from build123d import *

# Parameters (mm, degrees)
SKETCH1_W           = 40
SKETCH1_H           = 40
BOSS_EXTRUDE1_DEPTH = 5
SKETCH2_W           = 60
SKETCH2_H           = 60
BOSS_EXTRUDE2_DEPTH = 5
SKETCH3_R           = 7.5
BOSS_EXTRUDE3_DEPTH = 30
SKETCH4_W           = 30
SKETCH4_H           = 24
BOSS_EXTRUDE5_DEPTH = 10
FILLET1_R           = 5


with BuildPart() as part:
    # Sketch1 → Boss-Extrude1 (new body)
    with BuildSketch(Plane(origin=(0, 0, 0), x_dir=(1, 0, 0), z_dir=(0, 1, 0))):
        with Locations((20, 20)):
            Rectangle(SKETCH1_W, SKETCH1_H)
    extrude(amount=BOSS_EXTRUDE1_DEPTH)

    # Sketch2 → Boss-Extrude2 (add)
    with BuildSketch(Plane(origin=(0, 0, 0), x_dir=(-1, 0, 0), z_dir=(0, -1, 0))):
        with Locations((-20, 20)):
            Rectangle(SKETCH2_W, SKETCH2_H)
    extrude(amount=BOSS_EXTRUDE2_DEPTH)

    # Sketch3 → Boss-Extrude3 (add)
    with BuildSketch(Plane(origin=(0, -5, 0), x_dir=(-1, 0, 0), z_dir=(0, -1, 0))):
        with Locations(Location((-20, 5, 0), (0, 0, 90))):
            Circle(SKETCH3_R)
        with Locations(Location((-20, 35, 0), (0, 0, 90))):
            Circle(SKETCH3_R)
    extrude(amount=BOSS_EXTRUDE3_DEPTH)

    # Sketch4 → Boss-Extrude5 (add)
    with BuildSketch(Plane(origin=(0, -35, 0), x_dir=(-1, 0, 0), z_dir=(0, -1, 0))):
        with Locations((-25, 5)):
            Rectangle(SKETCH4_W, SKETCH4_H)
        with Locations((-25, 35)):
            Rectangle(SKETCH4_W, SKETCH4_H)
    extrude(amount=-BOSS_EXTRUDE5_DEPTH)

    # Fillet1
    fillet1_edges = [part.edges().sort_by_distance(p)[0] for p in [
        (40, -30, 7),
        (40, -30, -17),
        (10, -30, -17),
        (10, -30, 7),
        (40, -30, -23),
        (40, -30, -47),
        (10, -30, -47),
        (10, -30, -23),
    ]]
    fillet(fillet1_edges, radius=FILLET1_R)


solid = part.part
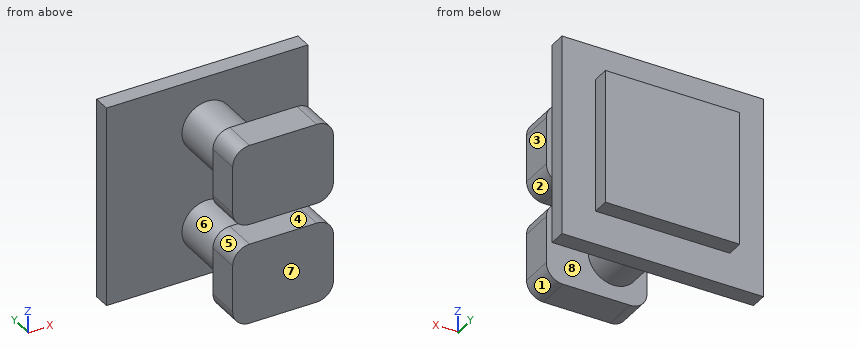
Design review of the part built by this model. Coordinates are the model's own, in mm. Face numbers are marked on the shaded views. A direction names the side the tool comes from. Round coordinates to 2 decimals unless told otherwise and drop trailing zeros. Write each loop counter-clockwise with the first axis right and the second up, starting at its lowest first coordinate (ties: lowest second). Pieces come first, ordered by that corner, then holes. Notation, with made-up numbers: (15.5, 7) -> (40.5, 7) arc R32 cw to (40.5, 38) -> close; hole circle Ø3 at (1.25, 72). An arc over 180 degrees is marked (long way). One line per question, with ' | ' between items.
(1) Insertion check: P1, Ø6, axis at x = -1.5, z = -3.5, coming from the +Y side; P2, Ø11, axis at x = 28, y = -31.5, coming from the +Z side; P3, Ø11, axis at y = -28, z = -4, coming from the +X side; P4, Ø3, axis at x = 20.5, y = -32, coming from the -Z side. Each pin has a flat end and moves straight along its axis. Give the tip position at first contact, or say it passes through.
Result sheet:
P1: y = 5 | P2: z = 7 | P3: x = 40 | P4: z = -47
(2) Take a section at B-B, the plane z = 6. State the section outline as (x, y) points.
Result sheet:
outline: (-10, -5) -> (50, -5) -> (50, 0) -> (-10, 0) -> close; (12, -35) -> (38, -35) -> (38, -25) -> (12, -25) -> close
(3) Draft analysis for pull direction Y (two halves, no side actions). For the marked faces 5, 6, 7 and 8, state which applies: released by +Y, released by -Y, zero draft, split by the parting line, or undercut.
Result sheet:
face 5: zero draft | face 6: undercut | face 7: released by -Y | face 8: undercut
(4) Take a section at C-C, the plane y = -27. State the section outline as (x, z) points, and give its area (3 significant figures).
Result sheet:
outline: (10, -42) arc R5 ccw to (15, -47) -> (35, -47) arc R5 ccw to (40, -42) -> (40, -28) arc R5 ccw to (35, -23) -> (15, -23) arc R5 ccw to (10, -28) -> close; (10, -12) arc R5 ccw to (15, -17) -> (35, -17) arc R5 ccw to (40, -12) -> (40, 2) arc R5 ccw to (35, 7) -> (15, 7) arc R5 ccw to (10, 2) -> close | area: 1,400 mm2
(5) Take a section at A-A, the plane x = 39. State the section outline as (y, z) points.
Result sheet:
outline: (-35, -45) -> (-25, -45) -> (-25, -25) -> (-35, -25) -> close; (-35, -15) -> (-25, -15) -> (-25, 5) -> (-35, 5) -> close; (-5, -50) -> (0, -50) -> (0, -40) -> (5, -40) -> (5, 0) -> (0, 0) -> (0, 10) -> (-5, 10) -> close
(6) Wall thickness on line 1 (Z direction, x = 20.5, y = -12); line 2 (Y direction, x = 12, z = -45); line 3 (Y direction, x = 28.5, z = -37.5): over which ranges is each line inside the solid? List them lowest first. Write a range as [from, to].
Result sheet:
line 1: [-42.48, -27.52], [-12.48, 2.48] | line 2: [-35, -25], [-5, 0] | line 3: [-35, -25], [-5, 5]
(7) Take a section at D-D, the plane x = 20. State the section outline as (y, z) points, and give its area (3 significant figures).
Result sheet:
outline: (-35, -47) -> (-25, -47) -> (-25, -42.5) -> (-5, -42.5) -> (-5, -50) -> (0, -50) -> (0, -40) -> (5, -40) -> (5, 0) -> (0, 0) -> (0, 10) -> (-5, 10) -> (-5, 2.5) -> (-25, 2.5) -> (-25, 7) -> (-35, 7) -> (-35, -17) -> (-25, -17) -> (-25, -12.5) -> (-5, -12.5) -> (-5, -27.5) -> (-25, -27.5) -> (-25, -23) -> (-35, -23) -> close | area: 1,580 mm2
(8) Machinability: for the marked faces 1, 2, 3 and 4, which of the approach directions +Z, -Z, +X, -X, +Y, -Y give a long, thin tool a straight path to every point of the face, cutting with its end or side? Answer none if there is none.
Result sheet:
face 1: -Z, +X, -Y | face 2: +X, -Y | face 3: +Z, -Z, +X, -Y | face 4: +X, -X, -Y
